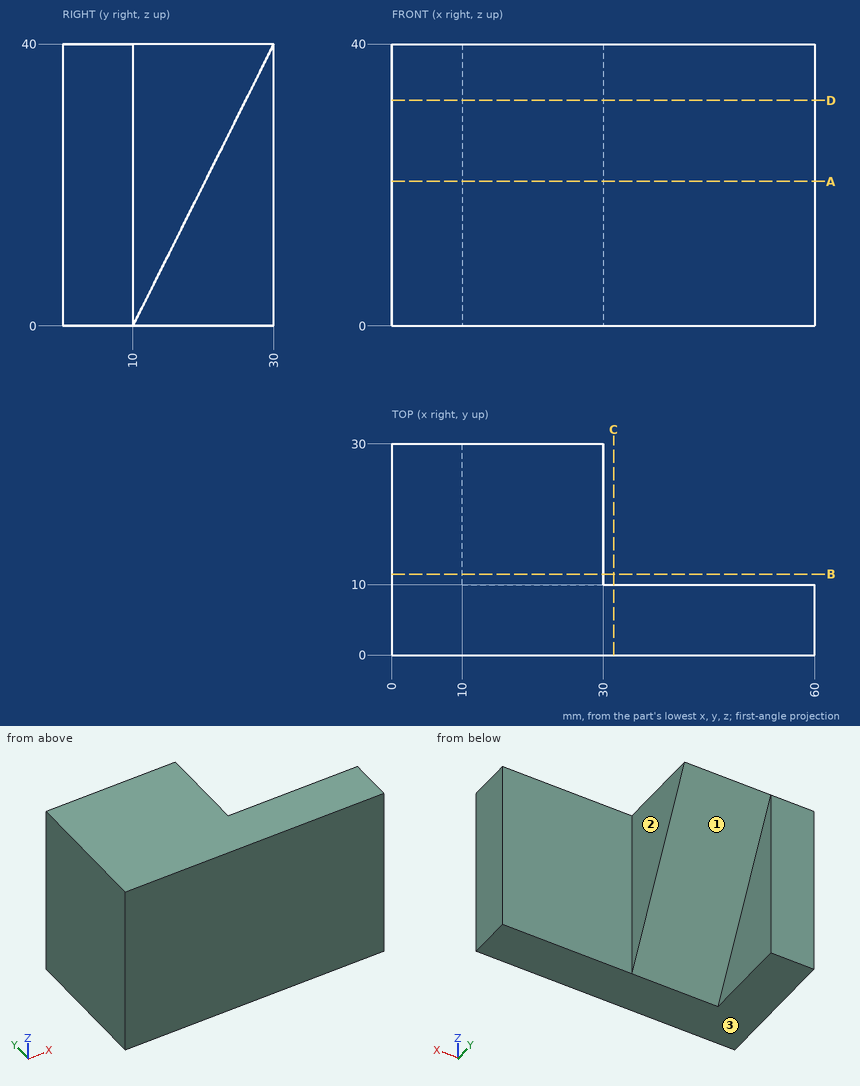
Drawing for the job (mm, zero at the part's lowest x, y, z). A direction names the side the tool comes from. Coordinates: 2 decimals unless noted, no trailing zeros. Order: outer loops, then holes, each group sorted by start corner. A loop starts at its lowest first (then second) coordinate and runs counter-clockwise, first axis right, second up.
Item 1: Band-saw the part on B-B on y = 11.5. List the corners of the cut face in (x, z).
Check sheet entries:
outline: (0, 0) - (10, 0) - (10, 3) - (30, 3) - (30, 40) - (0, 40) - close
Item 2: Band-saw the part on C-C on x = 31.5. List the corners of the cut face in (y, z).
Check sheet entries:
outline: (0, 0) - (10, 0) - (10, 40) - (0, 40) - close
Item 3: 3-axis set-ups, long thin cutter, end or side, ignore diameter. For the marked faces 1, 2 and 3: which of +Z, -Z, +X, -X, +Y, -Y reach the whole face in a straight line?
Check sheet entries:
face 1: -Z, +X, +Y
face 2: +Z, -Z, +X, +Y
face 3: -Z, +X, -X, +Y, -Y
Item 4: Drill centre lines: L1, parallel to X at y = 21, z = 11; L2, parallel to X at y = 14.5, z = 29. Where is each one in solid material? Low to high.
Check sheet entries:
L1: x = 0 to 10
L2: x = 0 to 30
Item 5: Pin check, flat tips, straight feed: pin 1 Ø1.5 at (y, z) = (24.5, 5) entering from +X; pin 2 Ø15 at (x, z) = (45.5, 17) entering from +Y; pin 3 Ø8 at (y, z) = (25.5, 23) entering from -X; pin 4 Ø8 at (x, z) = (31.5, 17) entering from +Y. Stop position of each tip, or through.
Check sheet entries:
pin 1: stops at x = 10
pin 2: stops at y = 10
pin 3: stops at x = 0
pin 4: stops at y = 20.35
Item 6: Band-saw the part on D-D on z = 32. List the corners of the cut face in (x, y), plus the area to 3 significant figures.
Check sheet entries:
outline: (0, 0) - (60, 0) - (60, 10) - (30, 10) - (30, 26) - (10, 26) - (10, 30) - (0, 30) - close
area: 1,120 mm2
Item 7: Band-saw the part on A-A on z = 20.5. List the corners of the cut face in (x, y).
Check sheet entries:
outline: (0, 0) - (60, 0) - (60, 10) - (30, 10) - (30, 20.25) - (10, 20.25) - (10, 30) - (0, 30) - close
